Autodesk Inventor part; units mm, degrees
ref_plane "YZ Plane" through (0, 0, 0) normal (1, 0, 0) x (0, 1, 0)
ref_plane "XZ Plane" through (0, 0, 0) normal (0, 1, 0) x (-1, 0, 0)
ref_plane "XY Plane" through (0, 0, 0) normal (0, 0, 1) x (1, 0, 0)
sketch "Sketch1" plane through (0, 0, 0) normal (0, 1, 0) x (-1, 0, 0)
  line L0 (3.0162, -25.0369) -> (-3.2338, -25.0369)
  line L1 (3.0162, -25.0369) -> (3.0162, 16.9631)
  line L2 (3.0162, 16.9631) -> (-3.2338, 16.9631)
  line L3 (-3.2338, 16.9631) -> (-3.2338, -25.0369)
  point P0 (0, 0)
  dimension "d1" = 6.25
  dimension "d3" = 42
extrude "Extrusion1" add sketch "Sketch1" along normal blind 4
sketch "Sketch10" plane through (3.2338, 0, -25.0369) normal (0, 0, -1) x (-1, 0, 0)
  circle A0 centre (3.2338, 1.4878) radius 1.2786
  point P0 (3.2338, 0)
sketch "Sketch12" plane through (0, 0, 0) normal (1, 0, 0) x (0, 1, 0)
  line L0 (0, -25.0369) -> (4, -25.0369)
  line L1 (2, -25.0369) -> (2, -33.0369)
  line L2 (0, -35.0369) -> (-6, -35.0369)
  line L3 (-8, -37.0369) -> (-8, -45.0369)
  arc A0 (0, -35.0369) -> (2, -33.0369) centre (0, -33.0369) ccw
  arc A1 (-6, -35.0369) -> (-8, -37.0369) centre (-6, -37.0369) ccw
  point P0 (0, 0)
  point P1 (2, -35.0369)
  point P2 (-8, -35.0369)
  dimension "d15" = 10
  dimension "d16" = 10
  dimension "d17" = 10
  dimension "d18" = 2
sweep "Sweep1" add profiles "Sketch10" path "Sketch12" path curves L1 A0 L2 A1 L3
sketch "Sketch14" plane through (0, 4, 0) normal (0, 1, 0) x (1, 0, 0)
  circle A0 centre (0, 3.2271) radius 2.25
  circle A1 centre (0, 16.2844) radius 2.25
  circle A2 centre (0, -10.1533) radius 2.25
  point P0 (0, 0)
  dimension "d29" = 4.5
  dimension "d30" = 4.5
  dimension "d31" = 4.5
extrude "Extrusion5" cut sketch "Sketch14" against normal blind 3.2
properties part number "Slits"
Input: part model. Units: mm. Frame: model coordinates. A direction names the side the tool comes from. Coordinates: 2 decimals unless noted, no trailing zeros. Loops run counter-clockwise (first coordinate to the right, second up) from the corner with the lowest first, then second, coordinate; pieces in that order, holes last.
Q1. Set-up query: faces 1 (the face through (0.166, 2.756, -29.093)), 2 (the face through (0, 0, -4)), 3 (the face through (-0.49, 2.42, -1.03)). Return all of +Z, -Z, +X, -X, +Y, -Y with unobstructed straight access to the full face (end or side cutting, diameter ignored); none if empty.
Q2. Cut plane D-D (z = -29). Output: boundary loops of the cut face in (x, y).
Q3. Material intervals for line 1 (Z direction, x = 0, y = 3.05); line 2 (Z direction, x = 0, y = 1.7); line 3 (Y direction, x = 2.75, z = -1), sorted ascending.
Q4. Contact query for flat-ended pins moving along their axis: pin 1 (3 mm diameter, centred on x = 0.5, y = 2, fed in from -Z); pin 2 (2 mm diameter, centred on x = 0.5, z = 9.5, fed in from +Y); pin 3 (2 mm diameter, centred on x = 0, y = -8, fed in from +Z). Output: stop coordinate, or through.
Q5. Cut plane B-B (z = -2). Output: boundary loops of the cut face in (x, y).
Q6. Cut plane C-C (y = -0.75). Output: boundary loops of the cut face in (x, z), then the cut area to 3 significant figures.
Q7. Cut plane A-A (x = 0). Output: boundary loops of the cut face in (y, z).
Q8. Draft query along Z for faces 4 (the face through (0.166, -7.244, -41.093)), 5 (the face through (0, 0.8, 10)), 6 (the face through (0.17, -3.04, -35.79)). Return one class per face: +Z half, -Z half, draft (parallel to the pull), parting line (faces both ways), or undercut.
Working result:
1. face 1: none
1. face 2: +Z, +X, -X, -Y
1. face 3: +Y
2. outline: circle Ø2.56 at (0, 1.49)
3. line 1: z = -25.04 to -18.53, -14.03 to -5.48, -0.98 to 7.9, 12.4 to 16.96
3. line 2: z = -35.22 to -18.53, -14.03 to -5.48, -0.98 to 7.9, 12.4 to 16.96
3. line 3: y = 0 to 4
4. pin 1: stops at z = -35.74
4. pin 2: stops at y = 0.8
4. pin 3: stops at z = -33.38
5. outline: (-3.02, 0) - (3.23, 0) - (3.23, 4) - (1.89, 4) - (1.89, 0.8) - (-1.89, 0.8) - (-1.89, 4) - (-3.02, 4) - close
6. outline: circle Ø2.56 at (0, -34.52)
6. area: 5.14 mm2
7. outline: (-9.79, -45.04) - (-7.23, -45.04) - (-7.23, -37.04) arc R1.23 cw to (-6, -35.8) - (0, -35.8) arc R2.77 ccw to (2.77, -33.04) - (2.77, -25.04) - (4, -25.04) - (4, -18.53) - (0.8, -18.53) - (0.8, -14.03) - (4, -14.03) - (4, -5.48) - (0.8, -5.48) - (0.8, -0.98) - (4, -0.98) - (4, 7.9) - (0.8, 7.9) - (0.8, 12.4) - (4, 12.4) - (4, 16.96) - (0, 16.96) - (0, -25.04) - (0.21, -25.04) - (0.21, -33.04) arc R0.21 cw to (0, -33.25) - (-6, -33.25) arc R3.79 ccw to (-9.79, -37.04) - close
8. face 4: draft
8. face 5: undercut
8. face 6: parting line
